from build123d import *

# Parameters (mm, degrees)
PAD_DEPTH              = 2
POCKET_DEPTH           = 0.08
POCKET001_DEPTH        = 0.08
SKETCH003_W            = 1.9
SKETCH003_H            = 6.6
POCKET002_DEPTH        = 0.55
LINEARPATTERN_COUNT    = 8
LINEARPATTERN_PITCH    = 2.378571
SKETCH004_W            = 2
SKETCH004_H            = 8.6
POCKET003_DEPTH        = 0.55
SKETCH005_W            = 1.9
SKETCH005_H            = 4.9
PAD001_DEPTH           = 0.1
LINEARPATTERN001_COUNT = 8
LINEARPATTERN001_PITCH = 2.378571
PAD002_DEPTH           = 0.1
POCKET004_DEPTH        = 111.893571
SKETCH008_W            = 7
SKETCH008_H            = 0.5
POCKET007_DEPTH        = 0.5
FILLET_R               = 0.6


with BuildPart() as part:
    # Sketch → Pad (new body)
    with BuildSketch(Plane.XY):
        Polygon((-12.021781, 15.95), (7.978219, 15.95), (12.021781, 11.906439), (12.021781, 6.25), (11.371781, 6.25), (11.371781, 4.55), (12.021781, 4.55), (12.021781, -15.95), (3.3, -15.95), (3.1, -15.75), (-3.1, -15.75), (-3.3, -15.95), (-12.021781, -15.95), (-12.021781, 1.35), (-11.221781, 1.35), (-11.221781, 8.35), (-12.021781, 8.35), align=None)
    extrude(amount=PAD_DEPTH)

    # Sketch001 → Pocket (cut)
    with BuildSketch(Plane.XY.offset(2)):
        with BuildLine():
            Line((-9.15, 12.15), (9.15, 12.15))
            ThreePointArc((10.15, 11.15), (9.857107, 11.857107), (9.15, 12.15))
            Line((10.15, 11.15), (10.15, -12.85))
            ThreePointArc((9.15, -13.85), (9.857107, -13.557107), (10.15, -12.85))
            Line((9.15, -13.85), (-9.15, -13.85))
            ThreePointArc((-10.15, -12.85), (-9.857107, -13.557107), (-9.15, -13.85))
            Line((-10.15, -12.85), (-10.15, 11.15))
            ThreePointArc((-9.15, 12.15), (-9.857107, 11.857107), (-10.15, 11.15))
        make_face()
    extrude(amount=-POCKET_DEPTH, mode=Mode.SUBTRACT)

    # Sketch002 → Pocket001 (cut)
    with BuildSketch(Plane.XY.offset(2)):
        with BuildLine():
            ThreePointArc((-7.35, -14.49), (-7.7, -14.84), (-7.35, -15.19))
            Line((-7.35, -15.19), (7.35, -15.19))
            ThreePointArc((7.35, -15.19), (7.7, -14.84), (7.35, -14.49))
            Line((-7.35, -14.49), (7.35, -14.49))
        make_face()
    extrude(amount=-POCKET001_DEPTH, mode=Mode.SUBTRACT)

    # Sketch003 → Pocket002 (cut)
    with BuildSketch(Plane(origin=(0, 0, 0), x_dir=(1, 0, 0), z_dir=(0, 0, -1))):
        with Locations((7.028219, -13.65)):
            Rectangle(SKETCH003_W, SKETCH003_H)
    pocket002 = extrude(amount=-POCKET002_DEPTH, mode=Mode.SUBTRACT)

    # LinearPattern: Pocket002 ×8
    with Locations(*[(-i * LINEARPATTERN_PITCH, 0, 0) for i in range(1, LINEARPATTERN_COUNT)]):
        add(pocket002, mode=Mode.SUBTRACT)

    # Sketch004 → Pocket003 (cut)
    with BuildSketch(Plane(origin=(0, 0, 0), x_dir=(1, 0, 0), z_dir=(0, 0, -1))):
        with Locations((9.678219, -12.65)):
            Rectangle(SKETCH004_W, SKETCH004_H)
    extrude(amount=-POCKET003_DEPTH, mode=Mode.SUBTRACT)

    # Sketch005 → Pad001 (new body)
    with BuildSketch(Plane(origin=(0, 0, 0.55), x_dir=(1, 0, 0), z_dir=(0, 0, -1))):
        with Locations((7.028219, -12.8)):
            Rectangle(SKETCH005_W, SKETCH005_H)
    pad001 = extrude(amount=PAD001_DEPTH)

    # LinearPattern001: Pad001 ×8
    with Locations(*[(-i * LINEARPATTERN001_PITCH, 0, 0) for i in range(1, LINEARPATTERN001_COUNT)]):
        add(pad001)

    # Sketch006 → Pad002 (new body)
    with BuildSketch(Plane(origin=(0, 0, 0.55), x_dir=(1, 0, 0), z_dir=(0, 0, -1))):
        Polygon((8.678219, -8.35), (8.678219, -13.15), (10.17822, -13.15), (10.678219, -12.650001), (10.678219, -8.35), align=None)
    extrude(amount=PAD002_DEPTH)

    # Sketch007 → Pocket004 (cut, through all)
    with BuildSketch(Plane.XZ.offset(15.95)):
        Polygon((-11.221781, 0.74), (-11.221781, -0.191555), (-12.614112, -0.191555), (-12.614112, 0), (-12.614112, 0.74), (-12.021781, 0.74), align=None)
    pocket004 = extrude(amount=-POCKET004_DEPTH, mode=Mode.SUBTRACT)

    # Mirrored: Pocket004 across Sketch007 V_Axis
    add(pocket004.mirror(Plane(origin=(0, -15.95, 0), x_dir=(0, -1, 0), z_dir=(1, 0, 0))), mode=Mode.SUBTRACT)

    # Sketch008 → Pocket007 (cut)
    with BuildSketch(Plane(origin=(-11.221781, 0, 0), x_dir=(0, -1, 0), z_dir=(-1, 0, 0))):
        with Locations((-4.85, 1.45)):
            Rectangle(SKETCH008_W, SKETCH008_H)
    extrude(amount=-POCKET007_DEPTH, mode=Mode.SUBTRACT)

    # Fillet
    fillet_edges = [part.edges().sort_by_distance(p)[0] for p in [
        (-12.021781, -15.95, 1.37),
        (-11.221781, -15.95, 0.37),
        (-12.021781, 15.95, 1.37),
        (11.221781, -15.95, 0.37),
        (12.021781, -15.95, 1.37),
        (-11.221781, 15.95, 0.37),
    ]]
    fillet(fillet_edges, radius=FILLET_R)


solid = part.part
Verification items for the finished model (mm, model axes). A direction names the side the tool comes from. Give positions to 0.01 mm unless a question says otherwise; leave off trailing zeros. Write each loop counter-clockwise with the first axis right and the second up, starting at its lowest first coordinate (ties: lowest second). Pieces come first, ordered by that corner, then holes. Notation, with made-up numbers: (-27.5, 45.25) -> (-3.5, 45.25) arc R15 ccw to (-3.5, 73.25) -> close; hole circle Ø1 at (14, 41.5). An arc over 180 degrees is marked (long way). Use CSV: the item, a comma, the result in double quotes.
(1) Sectioned sample at D-D (x = -9.75). Record the cut outline in (y, z).
Derived:
outline,"(-15.95, 0) -> (10.35, 0) -> (10.35, 0.45) -> (15.25, 0.45) -> (15.25, 0.55) -> (15.95, 0.55) -> (15.95, 2) -> (11.95, 2) -> (11.95, 1.92) -> (-13.65, 1.92) -> (-13.65, 2) -> (-15.95, 2) -> close"
(2) Set-up check for faces 4 (the flat face through (0, -15.75, 1)), 5 (the flat face through (11.372, 5, 1)), 6 (the flat face through (5, 13, 0.45)): record each of +Z, -Z, +X, -X, +Y, -Y from which the full face is reachable in a straight line by a thin tool's end or side.
Derived:
face 4,"+Z, -Z, -Y"
face 5,"+Z, -Z, +X"
face 6,"-Z, +Y"
(3) Sectioned sample at B-B (y = 5). Record the cut outline in (x, z).
Derived:
outline,"(-11.22, 0) -> (11.22, 0) -> (11.22, 0.74) -> (11.37, 0.74) -> (11.37, 2) -> (10.15, 2) -> (10.15, 1.92) -> (-10.15, 1.92) -> (-10.15, 2) -> (-11.22, 2) -> (-11.22, 1.7) -> (-10.72, 1.7) -> (-10.72, 1.2) -> (-11.22, 1.2) -> close"
(4) Material ranges on L1, parallel to Z at x = -0.75, y = 5; L2, parallel to X at y = 2.5, z = 0.5; L3, parallel to Y at x = 2.75, z = 0.4, recorded low to high.
Derived:
L1,"z = 0 to 1.92"
L2,"x = -11.22 to 11.22"
L3,"y = -15.75 to 10.35"
(5) Sectioned sample at A-A (x = 4.5). Record the cut outline in (y, z), plus the area to 3 significant figures.
Derived:
outline,"(-15.95, 0) -> (10.35, 0) -> (10.35, 0.45) -> (15.25, 0.45) -> (15.25, 0.55) -> (15.95, 0.55) -> (15.95, 2) -> (12.15, 2) -> (12.15, 1.92) -> (-13.85, 1.92) -> (-13.85, 2) -> (-14.49, 2) -> (-14.49, 1.92) -> (-15.19, 1.92) -> (-15.19, 2) -> (-15.95, 2) -> close"
area,"59.1 mm^2"
(6) Go/stop test with flat-tipped pins: pin 1 (0.6 mm diameter, centred on y = 13, z = 0.5, fed in from -X); pin 2 (6 mm diameter, centred on x = 0, y = -2, fed in from +Z); pin 3 (1.5 mm diameter, centred on x = 0, y = 12.5, fed in from -Z). Record where each tip stops, or that it passes through.
Derived:
pin 1,"stops at x = -12.02"
pin 2,"stops at z = 1.92"
pin 3,"stops at z = 0.45"
(7) Release check for a two-part mould opening along Y. For faces 1 (the flat face through (-11.5, 8.35, 1.4)), 2 (the flat face through (11.6, -1.8, 0.74)), 3 (the flat face through (7, -15.95, 1)) record: +Y half, -Y half, draft (parallel to the pull), parting line (faces both ways), or undercut.
Derived:
face 1,"undercut"
face 2,"draft"
face 3,"-Y half"
(8) Sectioned sample at C-C (y = -14.84). Record the cut outline in (x, z), plus the area to 3 significant figures.
Derived:
outline,"(-12.02, 0.74) -> (-11.22, 0.74) -> (-11.22, 0) -> (11.22, 0) -> (11.22, 0.74) -> (12.02, 0.74) -> (12.02, 2) -> (7.7, 2) -> (7.7, 1.92) -> (-7.7, 1.92) -> (-7.7, 2) -> (-12.02, 2) -> close"
area,"45.7 mm^2"
